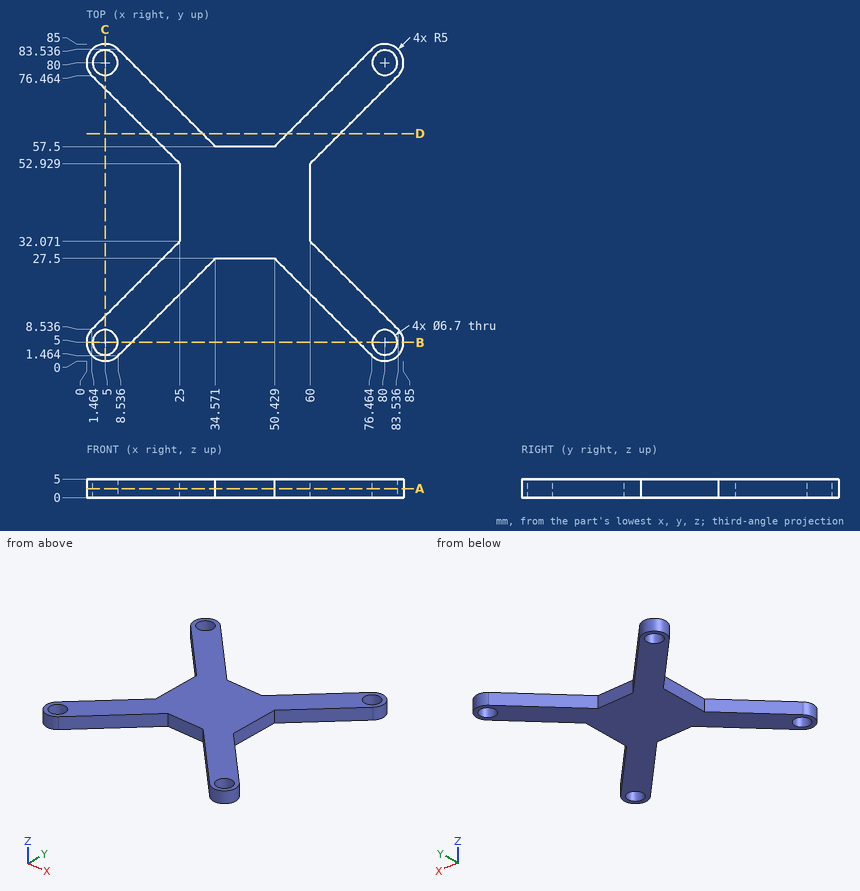
Here's the drawing with two shaded views (mm, measured from the low corner). I have some questions. Coordinates: 2 decimals unless noted, no trailing zeros. Order: outer loops, then holes, each group sorted by start corner. A loop starts at its lowest first (then second) coordinate and runs counter-clockwise, first axis right, second up.
Item 1: If we section it at A-A, the plane z = 2.45: Give the number of separate pieces and of enclosed holes in the cut face, then the cut area to 3 significant figures.
Response values:
separate pieces: 1
enclosed holes: 4
area: 2,380 mm2
Item 2: If we section it at B-B, the plane y = 5: List the corners of the cut face in (x, z) for me.
Response values:
outline: (0, 0) - (1.65, 0) - (1.65, 5) - (0, 5) - close; (8.35, 0) - (12.07, 0) - (12.07, 5) - (8.35, 5) - close; (72.93, 0) - (76.65, 0) - (76.65, 5) - (72.93, 5) - close; (83.35, 0) - (85, 0) - (85, 5) - (83.35, 5) - close
Item 3: I'm going to push flat-ended pins straight in: pin 1 Ø5.5 at (x, y) = (5, 5) entering from +Z; pin 2 Ø3 at (y, z) = (75, 1.5) entering from +X; pin 3 Ø2.5 at (x, z) = (43, 1.5) entering from +Y. Where does each tip first touch, or does it pass through?
Response values:
pin 1: passes through
pin 2: stops at x = 83.57
pin 3: stops at y = 57.5
Item 4: I need wall thicknesses on probe 1 along Y at (x, z) = (5, 2.15); probe 2 along X at (y, z) = (81.5, 0.85) (1 decimal); probe 3 along Y at (x, z) = (77, 4.1) (1 decimal). Which ranges of each line are inside material? Lowest first, please.
Response values:
probe 1: y = 0 to 1.65, 8.35 to 12.07, 72.93 to 76.65, 83.35 to 85
probe 2: x = 0.2 to 2, 8 to 10.6, 74.4 to 77, 83 to 84.8
probe 3: y = 1 to 3.5, 6.5 to 15.1, 69.9 to 78.5, 81.5 to 84
Item 5: If we section it at D-D, the plane y = 61: List the corners of the cut face in (x, z) for me, then the cut area to 3 significant figures.
Response values:
outline: (16.93, 0) - (31.07, 0) - (31.07, 5) - (16.93, 5) - close; (53.93, 0) - (68.07, 0) - (68.07, 5) - (53.93, 5) - close
area: 141 mm2
